Answer from the drawing. Dimensions are ordinates in mm from the lowest x, y and z of the part. Give positions to 0.01 mm unless a question says otherwise; leave off trailing zeros. Loops run counter-clockwise (first coordinate to the right, second up) from the corner with the lowest first, then second, coordinate; pieces in that order, holes last.
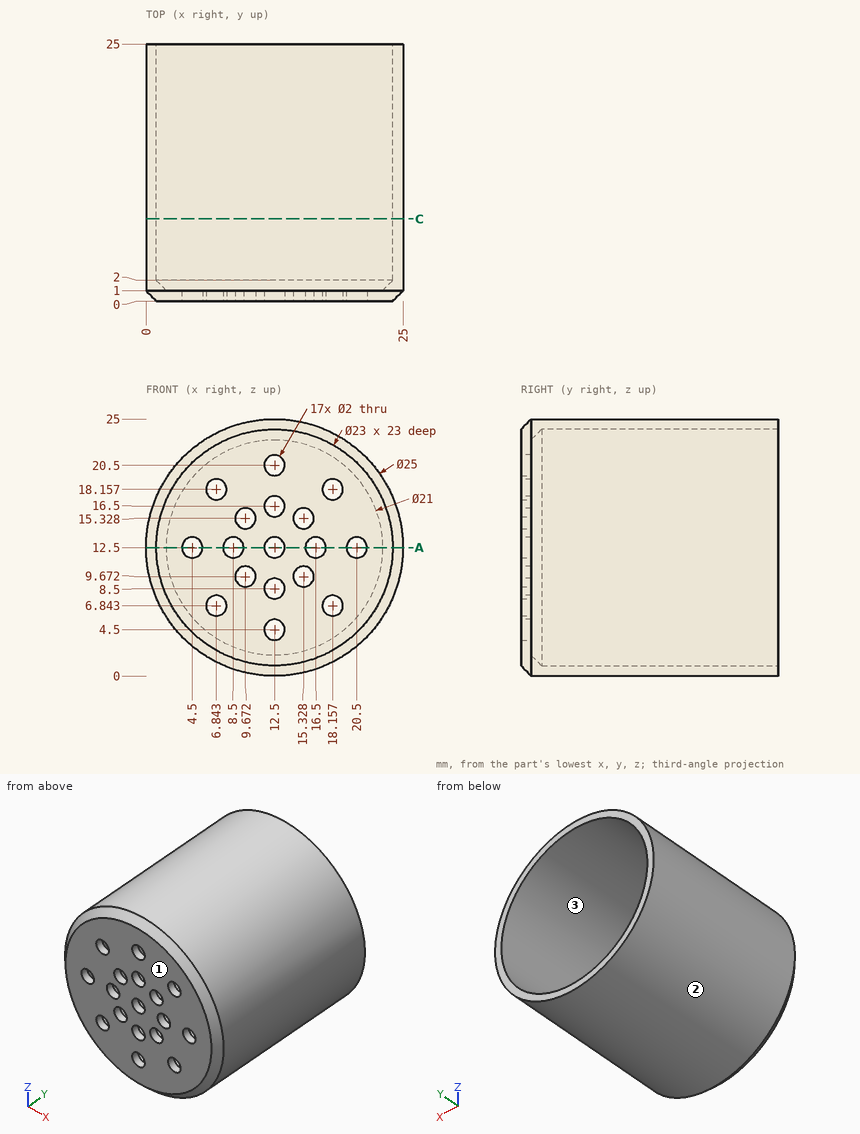
Item 1: Flat-ended cylindrical pins translate along their axes: pin 1 Ø2.5 at (x, z) = (12.5, 20.5) entering from +Y; pin 2 Ø1.6 at (x, z) = (12.5, 16.5) entering from +Y; pin 3 Ø10 at (y, z) = (19, 18.5) entering from +X; pin 4 Ø1 at (x, y) = (9, 9.5) entering from +Z (1 decimal). Find the tip coordinate at first contact, or state that the pin passes through.
Item 2: Determine the mould class of the marked faces 1, 2 and 3 for opening direction X: released by +X, released by -X, zero draft, split by the parting line, or undercut.
Item 3: Consider line 1 (X direction, y = 0.3, z = 12.5); line 2 (Y direction, x = 4.5, z = 14.5); line 3 (Z direction, x = 3.5, y = 1.5) (1 decimal). Determine where each line is inside the solid, lowest interval first.
Item 4: Find section A-A, the plane z = 12.5. Give the number of separate pieces and of enclosed holes in the cut face.
Item 5: Find section C-C, the plane y = 8. Write down the section's boundary in (x, z).
Ans:
1. pin 1: stops at y = 1
1. pin 2: passes through
1. pin 3: stops at x = 24.96
1. pin 4: stops at z = 24.6
2. face 1: zero draft
2. face 2: split by the parting line
2. face 3: undercut
3. line 1: x = 0.7 to 3.5, 5.5 to 7.5, 9.5 to 11.5, 13.5 to 15.5, 17.5 to 19.5, 21.5 to 24.3
3. line 2: y = 0 to 1
3. line 3: z = 3.8 to 6.2, 18.8 to 21.2
4. separate pieces: 6
4. enclosed holes: 0
5. outline: circle Ø25 at (12.5, 12.5); hole circle Ø23 at (12.5, 12.5)
